```python
from build123d import *


with BuildPart() as part:
    # Sketch2 → Revolve1 (revolve)
    with BuildSketch(Plane.XY):
        with BuildLine():
            Line((0, -37.091298276), (32.5, -37.091298276))
            Line((32.5, -37.091298276), (11.66645179, -30.935726736))
            ThreePointArc((11.66645179, -30.935726736), (6.489523045, -27.331580559), (4.5, -21.345575301))
            Line((4.5, -21.345575301), (4.5, 10.145686892))
            ThreePointArc((4.5, 10.145686892), (6.311054798, 15.885127323), (11.088235294, 19.545679529))
            ThreePointArc((11.088235294, 19.545679529), (27.887861488, 33.406821561), (32.163132951, 54.762868775))
            Line((32.163132951, 54.762868775), (23, 117.908701724))
            Line((23, 117.908701724), (21.989526299, 117.908701724))
            Line((21.989526299, 117.908701724), (31.173498091, 54.619262216))
            ThreePointArc((31.173498091, 54.619262216), (23.819567674, 29.483081871), (0, 18.595655602))
            Line((0, 18.595655602), (0, -37.091298276))
        make_face()
    revolve(axis=Axis((0, 117.908701724, 0), (0, -1, 0)))


solid = part.part
```
Geometry check sheet. Reference: the model listing, model coordinates, mm. A direction names the side the tool comes from. Give positions to 0.01 mm unless a question says otherwise; leave off trailing zeros. Write each loop counter-clockwise with the first axis right and the second up, starting at its lowest first coordinate (ties: lowest second). Pieces come first, ordered by that corner, then holes.
1) Release check for a two-part mould opening along Y. For faces 1 (the conical face through (-5.74, 93.79, -25.87)), 2 (the flat face through (0, -37.091, 0)), 3 (the conical face through (-10.061, -31.235, -7.714)) record: pulls with the +Y half, pulls with the -Y half, needs draft (parallel to the pull), parting line crosses it, or undercut.
2) Material ranges on L1, parallel to X at y = 61, z = -25.5; L2, parallel to Z at x = 19, y = 54.5; L3, parallel to X at y = 63, z = 27.5, recorded low to high.
3) Section check A-A, the plane z = 25.5. State how many separate pieces and enclosed holes the cut face has, and give its area (3 significant figures).
4) Section check B-B, the plane x = 0. Record the boundary of the cut face in (y, z).
5) Access from +Z, -Z, +X, -X, +Y, -Y to the whole of each face (thin tool, end or side, straight path). Record for faces 4 (the cylindrical face through (-0.59, -5.38, 4.46)), 5 (the flat face through (12, 117.909, -19)).
6) Section check C-C, the plane y = 43.5. Record the boundary of the cut face in (x, z), and give its area (3 significant figures).
7) Section check D-D, the plane z = 0. Record the boundary of the cut face in (x, y).
8) Gauge pin test, flat ends, axial feed: pin 1 (12 mm diameter, centred on y = 17, z = -0.5, fed in from +X); pin 2 (12 mm diameter, centred on x = -7.5, y = 96.5, fed in from -Z); pin 3 (8 mm diameter, centred on y = 82, z = -16, fed in from +X). Record the tip position at first contact, or that the pin passes through.
Computed:
1. face 1: pulls with the +Y half
1. face 2: pulls with the -Y half
1. face 3: undercut
2. L1: x = -18.08 to -16.27, 16.27 to 18.08
2. L2: z = -26 to -24.74, 24.74 to 26
2. L3: x = -14.24 to -11.88, 11.88 to 14.24
3. separate pieces: 2
3. enclosed holes: 1
3. area: 432 mm2
4. outline: (-37.09, -32.5) - (-30.94, -11.67) arc R10 cw to (-21.35, -4.5) - (10.15, -4.5) arc R10 cw to (19.55, -11.09) arc R32.5 ccw to (54.76, -32.16) - (117.91, -23) - (117.91, -21.99) - (54.62, -31.17) arc R31.5 cw (long way) to (54.62, 31.17) - (117.91, 21.99) - (117.91, 23) - (54.76, 32.16) arc R32.5 ccw to (19.55, 11.09) arc R10 cw to (10.15, 4.5) - (-21.35, 4.5) arc R10 cw to (-30.94, 11.67) - (-37.09, 32.5) - close
5. face 4: none
5. face 5: +Z, -Z, +X, -X, +Y
6. outline: circle Ø63.65 at (0, 0); hole circle Ø61.6 at (0, 0)
6. area: 201 mm2
7. outline: (-32.5, -37.09) - (32.5, -37.09) - (11.67, -30.94) arc R10 cw to (4.5, -21.35) - (4.5, 10.15) arc R10 cw to (11.09, 19.55) arc R32.5 ccw to (32.16, 54.76) - (23, 117.91) - (21.99, 117.91) - (31.17, 54.62) arc R31.5 cw (long way) to (-31.17, 54.62) - (-21.99, 117.91) - (-23, 117.91) - (-32.16, 54.76) arc R32.5 ccw to (-11.09, 19.55) arc R10 cw to (-4.5, 10.15) - (-4.5, -21.35) arc R10 cw to (-11.67, -30.94) - close
8. pin 1: stops at x = 17.94
8. pin 2: stops at z = -26.53
8. pin 3: stops at x = 25.64
